Geometry: final body of the model. Coordinates: model frame, mm. Face numbers are marked on the shaded views. Round coordinates to 2 decimals unless told otherwise and drop trailing zeros. Loops run counter-clockwise (first coordinate to the right, second up) from the corner with the lowest first, then second, coordinate; pieces in that order, holes last. Notation, with made-up numbers: (20.25, -32.5) - (53.25, -32.5) arc R21 cw to (53.25, -15.5) - close; hole circle Ø2 at (-29, 50). An arc over 180 degrees is marked (long way). Answer as CSV lines item,"result".
from build123d import *

# Parameters (mm, degrees)
SKETCH1_R                   = 72.5
BOSS_EXTRUDE1_DEPTH         = 10
SKETCH1_3_R                 = 12.5
BOSS_EXTRUDE2_DEPTH         = 11.55
SKETCH1_4_R                 = 49.75
SKETCH1_4_R_2               = 37.75
BOSS_EXTRUDE3_DEPTH         = 6
BOSS_EXTRUDE4_START         = -13.8
SKETCH1_5_R                 = 72.5
SKETCH1_5_R_2               = 67.525
BOSS_EXTRUDE4_DEPTH         = 13.8
CUT_EXTRUDE1_REACH          = 111.771
CUT_EXTRUDE1_START          = -5
SKETCH2_R                   = 2.75
M3_TAPPED_HOLE1_D           = 2.5
M3_TAPPED_HOLE1_CSINK_D     = 3.05
M3_TAPPED_HOLE1_CSINK_ANGLE = 90
SKETCH6_R                   = 2.5
CUT_EXTRUDE2_DEPTH          = 6


with BuildPart() as part:
    # Sketch1 → Boss-Extrude1 (new body)
    with BuildSketch(Plane(origin=(0, 0, 0), x_dir=(0, 0, -1), z_dir=(1, 0, 0))):
        Circle(SKETCH1_R)
    extrude(amount=BOSS_EXTRUDE1_DEPTH)

    # Sketch1<3> → Boss-Extrude2 (add)
    with BuildSketch(Plane(origin=(0, 0, 0), x_dir=(0, 0, -1), z_dir=(1, 0, 0))):
        Circle(SKETCH1_3_R)
    extrude(amount=-BOSS_EXTRUDE2_DEPTH)

    # Sketch1<4> → Boss-Extrude3 (add)
    with BuildSketch(Plane(origin=(0, 0, 0), x_dir=(0, 0, -1), z_dir=(1, 0, 0))):
        Circle(SKETCH1_4_R)
        Circle(SKETCH1_4_R_2, mode=Mode.SUBTRACT)
    extrude(amount=-BOSS_EXTRUDE3_DEPTH)

    # Sketch1<5> → Boss-Extrude4 (add)
    with BuildSketch(Plane(origin=(0, 0, 0), x_dir=(0, 0, -1), z_dir=(1, 0, 0)).offset(BOSS_EXTRUDE4_START)):
        Circle(SKETCH1_5_R)
        Circle(SKETCH1_5_R_2, mode=Mode.SUBTRACT)
    extrude(amount=BOSS_EXTRUDE4_DEPTH)

    # Sketch2 → Cut-Extrude1 (cut, up to next)
    with BuildSketch(Plane.ZY.offset(11.55).offset(CUT_EXTRUDE1_START), mode=Mode.PRIVATE) as cut_extrude1_sk1:
        with Locations((0, 9)):
            Circle(SKETCH2_R)
    cut_extrude1_tool1 = extrude(cut_extrude1_sk1.sketch, amount=-CUT_EXTRUDE1_REACH, mode=Mode.PRIVATE) & part.part
    # Sketch2 → Cut-Extrude1 (cut, up to next)
    with BuildSketch(Plane.ZY.offset(11.55).offset(CUT_EXTRUDE1_START), mode=Mode.PRIVATE) as cut_extrude1_sk2:
        with Locations((7.794228634, 4.5)):
            Circle(SKETCH2_R)
    cut_extrude1_tool2 = extrude(cut_extrude1_sk2.sketch, amount=-CUT_EXTRUDE1_REACH, mode=Mode.PRIVATE) & part.part
    # Sketch2 → Cut-Extrude1 (cut, up to next)
    with BuildSketch(Plane.ZY.offset(11.55).offset(CUT_EXTRUDE1_START), mode=Mode.PRIVATE) as cut_extrude1_sk3:
        with Locations((7.794228634, -4.5)):
            Circle(SKETCH2_R)
    cut_extrude1_tool3 = extrude(cut_extrude1_sk3.sketch, amount=-CUT_EXTRUDE1_REACH, mode=Mode.PRIVATE) & part.part
    # Sketch2 → Cut-Extrude1 (cut, up to next)
    with BuildSketch(Plane.ZY.offset(11.55).offset(CUT_EXTRUDE1_START), mode=Mode.PRIVATE) as cut_extrude1_sk4:
        with Locations((0, -9)):
            Circle(SKETCH2_R)
    cut_extrude1_tool4 = extrude(cut_extrude1_sk4.sketch, amount=-CUT_EXTRUDE1_REACH, mode=Mode.PRIVATE) & part.part
    # Sketch2 → Cut-Extrude1 (cut, up to next)
    with BuildSketch(Plane.ZY.offset(11.55).offset(CUT_EXTRUDE1_START), mode=Mode.PRIVATE) as cut_extrude1_sk5:
        with Locations((-7.794228634, -4.5)):
            Circle(SKETCH2_R)
    cut_extrude1_tool5 = extrude(cut_extrude1_sk5.sketch, amount=-CUT_EXTRUDE1_REACH, mode=Mode.PRIVATE) & part.part
    # Sketch2 → Cut-Extrude1 (cut, up to next)
    with BuildSketch(Plane.ZY.offset(11.55).offset(CUT_EXTRUDE1_START), mode=Mode.PRIVATE) as cut_extrude1_sk6:
        with Locations((-7.794228634, 4.5)):
            Circle(SKETCH2_R)
    cut_extrude1_tool6 = extrude(cut_extrude1_sk6.sketch, amount=-CUT_EXTRUDE1_REACH, mode=Mode.PRIVATE) & part.part
    add(cut_extrude1_tool1.solids().sort_by_distance((-6.55, 9, 0))[0], mode=Mode.SUBTRACT)
    add(cut_extrude1_tool2.solids().sort_by_distance((-6.55, 4.5, 7.794229))[0], mode=Mode.SUBTRACT)
    add(cut_extrude1_tool3.solids().sort_by_distance((-6.55, -4.5, 7.794229))[0], mode=Mode.SUBTRACT)
    add(cut_extrude1_tool4.solids().sort_by_distance((-6.55, -9, 0))[0], mode=Mode.SUBTRACT)
    add(cut_extrude1_tool5.solids().sort_by_distance((-6.55, -4.5, -7.794229))[0], mode=Mode.SUBTRACT)
    add(cut_extrude1_tool6.solids().sort_by_distance((-6.55, 4.5, -7.794229))[0], mode=Mode.SUBTRACT)

    # M3 Tapped Hole1 (through all)
    with Locations(Plane.ZY.offset(11.55)):
        with Locations((0, 9), (7.794228634, 4.5), (7.794228634, -4.5), (0, -9), (-7.794228634, -4.5), (-7.794228634, 4.5)):
            CounterSinkHole(M3_TAPPED_HOLE1_D / 2, M3_TAPPED_HOLE1_CSINK_D / 2, counter_sink_angle=M3_TAPPED_HOLE1_CSINK_ANGLE)

    # Sketch6 → Cut-Extrude2 (cut)
    with BuildSketch(Plane(origin=(10, 0, 0), x_dir=(0, 0, -1), z_dir=(1, 0, 0))):
        with Locations((-62.5, 0)):
            Circle(SKETCH6_R)
        with Locations((-31.25, 54.126587737)):
            Circle(SKETCH6_R)
        with Locations((31.25, 54.126587737)):
            Circle(SKETCH6_R)
        with Locations((62.5, 0)):
            Circle(SKETCH6_R)
        with Locations((31.25, -54.126587737)):
            Circle(SKETCH6_R)
        with Locations((-31.25, -54.126587737)):
            Circle(SKETCH6_R)
    extrude(amount=-CUT_EXTRUDE2_DEPTH, mode=Mode.SUBTRACT)


solid = part.part
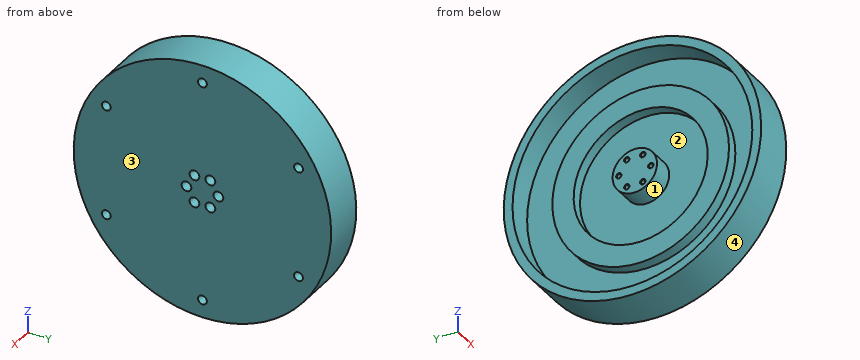
(1) Section D-D (z = 20). Output: boundary loops of the cut face in (x, y).
Findings below:
outline,"(-13.8, -69.69) - (10, -69.69) - (10, 69.69) - (-13.8, 69.69) - (-13.8, 64.5) - (0, 64.5) - (0, 45.55) - (-6, 45.55) - (-6, 32.02) - (0, 32.02) - (0, -32.02) - (-6, -32.02) - (-6, -45.55) - (0, -45.55) - (0, -64.5) - (-13.8, -64.5) - close"
(2) Section C-C (y = 40.5). Output: boundary loops of the cut face in (x, z).
Findings below:
outline,"(-13.8, -60.13) - (10, -60.13) - (10, 60.13) - (-13.8, 60.13) - (-13.8, 54.03) - (0, 54.03) - (0, 28.89) - (-6, 28.89) - (-6, -28.89) - (0, -28.89) - (0, -54.03) - (-13.8, -54.03) - close"
(3) Draft query along Z for the marked faces 1, 2, 3 and 4. Return one class per face: pulls with the +Z half, pulls with the -Z half, needs draft (parallel to the pull), parting line crosses it, or undercut.
Findings below:
face 1,"undercut"
face 2,"undercut"
face 3,"needs draft"
face 4,"parting line crosses it"
(4) Pin query (flat end, axial travel): P1, Ø4, axis at y = 4.5, z = 7.79, coming from the -X side; P2, Ø1.5, axis at x = 4, z = 47, coming from the -Y side; P3, Ø12, axis at x = -10.5, z = -54.5, coming from the -Y side. Return the tip coordinate at first contact, or that it passes through.
Findings below:
P1,"x = -11.55"
P2,"y = -55.83"
P3,"y = -53.89"
(5) Section A-A (x = -1.75). Give the number of separate pieces and of enclosed holes in the cut face, and give its area (3 significant figures).
Findings below:
separate pieces,"3"
enclosed holes,"8"
area,"5,840 mm2"
(6) Section B-B (z = 62). Output: boundary loops of the cut face in (x, y), and give its area (3 significant figures).
Findings below:
outline,"(-13.8, -37.58) - (10, -37.58) - (10, -2.45) - (4, -2.45) - (4, 2.45) - (10, 2.45) - (10, 37.58) - (-13.8, 37.58) - (-13.8, 26.75) - (0, 26.75) - (0, -26.75) - (-13.8, -26.75) - close"
area,"1,020 mm2"
(7) Material intervals for line 1 along Z through (x, y) = (-4.75, -16.5); line 2 along Z through (x, y) = (-3.75, -34); line 3 along Z through (x, y) = (4.25, -2), sorted ascending.
Findings below:
line 1,"-70.6 to -65.48, -46.93 to -33.95, 33.95 to 46.93, 65.48 to 70.6"
line 2,"-64.03 to -58.34, -36.32 to -16.4, 16.4 to 36.32, 58.34 to 64.03"
line 3,"-72.47 to -64, -61 to -8.94, -6.65 to 6.65, 8.94 to 61, 64 to 72.47"
